Autodesk Inventor part; units mm, degrees
ref_plane "XZ Plane" through (0, 0, 0) normal (0, 1, 0) x (-1, 0, 0)
ref_plane "XY Plane" through (0, 0, 0) normal (0, 0, 1) x (1, 0, 0)
sketch "Sketch1" plane through (0, 0, 0) normal (0, 1, 0) x (-1, 0, 0)
  line L0 (47.625, 50.8) -> (-47.625, 50.8)
  line L1 (-47.625, 50.8) -> (-47.625, -50.8)
  line L2 (-47.625, -50.8) -> (47.625, -50.8)
  line L3 (47.625, -50.8) -> (47.625, 50.8)
  line L4 (47.625, 50.8) -> (-47.625, -50.8) construction
  line L5 (-47.625, 50.8) -> (47.625, -50.8) construction
  point P0 (0, 0)
  dimension "d0" = 95.25
  dimension "d1" = 101.6
extrude "Extrusion1" add sketch "Sketch1" against normal blind 3.175
sketch "Sketch2" plane through (0, 0, 0) normal (0, 1, 0) x (1, 0, 0)
  line L0 (-47.625, -19.05) -> (-28.575, -19.05)
  line L1 (-28.575, -19.05) -> (-28.575, 19.05)
  line L2 (-28.575, 19.05) -> (-47.625, 19.05)
  line L3 (-47.625, 19.05) -> (-47.625, -19.05)
  line L4 (-47.625, -19.05) -> (-28.575, 19.05) construction
  line L5 (-28.575, -19.05) -> (-47.625, 19.05) construction
  line L6 (-44.45, -15.875) -> (-31.75, -15.875)
  line L7 (-31.75, -15.875) -> (-31.75, 15.875)
  line L8 (-31.75, 15.875) -> (-44.45, 15.875)
  line L9 (-44.45, 15.875) -> (-44.45, -15.875)
  line L10 (-44.45, -15.875) -> (-31.75, 15.875) construction
  line L11 (-31.75, -15.875) -> (-44.45, 15.875) construction
  line L12 (-47.625, 50.8) -> (47.625, 50.8) construction
  line L13 (0, 50.8) -> (0, -101.6) construction
  line L14 (47.625, -19.05) -> (28.575, -19.05)
  line L15 (28.575, -19.05) -> (28.575, 19.05)
  line L16 (28.575, 19.05) -> (47.625, 19.05)
  line L17 (47.625, 19.05) -> (47.625, -19.05)
  line L18 (44.45, -15.875) -> (31.75, -15.875)
  line L19 (31.75, -15.875) -> (31.75, 15.875)
  line L20 (31.75, 15.875) -> (44.45, 15.875)
  line L21 (44.45, 15.875) -> (44.45, -15.875)
  point P0 (0, 0)
  point P1 (-38.1, 0)
  dimension "d4" = 38.1
  dimension "d5" = 19.05
  dimension "d6" = 38.1
  dimension "d7" = 3.175
  dimension "d8" = 3.175
extrude "Extrusion2" add sketch "Sketch2" along normal blind 101.6
sketch "Sketch4" plane through (-47.625, -3.175, -50.8) normal (-1, 0, 0) x (0, 0, 1)
  line L0 (50.8, 3.175) -> (50.8, 93.283) construction
  circle A0 centre (50.8, 79.375) radius 4.7625
  line L1 (0, 3.175) -> (31.75, 3.175)
  dimension "d15" = 9.525
  dimension "d16" = 76.2
extrude "Extrusion4" cut sketch "Sketch4" against normal through all
equation "\"d0\" = BaseWidth"
equation "\"d1\" = BaseLength"
equation "\"d2\" = BaseThickness"
equation "\"d5\" = postWidth"
equation "\"d6\" = postLength"
equation "\"d7\" = postThickness"
equation "\"d8\" = postThickness"
equation "\"d9\" = postHeight"
equation "\"d15\" = axelDiam"
equation "\"d16\" = axelHeightAbovePlate"
equation "\"BaseWidth\" = 95.25"
equation "\"BaseLength\" = 101.6"
equation "\"BaseThickness\" = 3.175"
equation "\"postWidth\" = 19.05"
equation "\"postLength\" = 38.1"
equation "\"postThickness\" = 3.175"
equation "\"postCenterDistanceFromCenterOfBase\" = 38.1"
equation "\"axelDiam\" = 9.525"
equation "\"axelHeightAbovePlate\" = 76.2"
properties part number "PostForLift"
The listing builds one solid part. Answer for the finished solid, in the listing's coordinates (mm). A direction names the side the tool comes from. Coordinates: 2 decimals unless noted, no trailing zeros. Loops run counter-clockwise (first coordinate to the right, second up) from the corner with the lowest first, then second, coordinate; pieces in that order, holes last. Notation, with made-up numbers: M 45.5,-0.75 L 69.5,-0.75 A22 cw 69.5,16.25 Z; hole C -38.5,67.5 d10. An arc over 180 degrees is marked long. Answer as CSV lines item,"result". Start each with the question number.
(1) For faces 1 (the flat face through (-38, 50, 15.875)), 2 (the cylindrical face through (30.14, 80.92, -0.62)), 3 (the flat face through (-47.625, 42, 4)), 4 (the flat face through (-38, 50, 19.05)), 5 (the flat face through (-28.575, 50, 0)), determine the directions among +Z, -Z, +X, -X, +Y, -Y from which every point of the face is accessible in a straight line to the end or side of a thin tool.
(2) The part is cut by section B-B (z = 0). State how many separate pieces and enclosed holes the cut face has, and give its area (3 significant figures).
(3) Given pin 1 (2 mm diameter, centred on y = 7.5, z = -22, fed in from +X); pin 2 (6.5 mm diameter, centred on x = 38, z = 0, fed in from +Y); pin 3 (15 mm diameter, centred on x = 36.5, y = 63, fed in from +Z); pin 4 (15 mm diameter, centred on x = 37, y = 40, fed in from -Z), each flat-ended and moving along its own axis, determine where each tip first touches the part or whether it passes through.
(4) The part is cut by section D-D (x = 12). Give the vertices of the cut face in (y, z) (3 decimals), and give its area (3 significant figures).
(5) Find the intervals of material crossed by L1, parallel to X at y = 4.5, z = 12 (3 decimals); L2, parallel to Y at x = -30.7, z = 0 (1 decimal); L3, parallel to Z at x = -30, y = 76, in increasing order. Write a range as [from, to].
(6) The mould has two halves that part along Z. Classify faces 6 (the flat face through (38, 50, -19.05)), 7 (the flat face through (-38, 0, 0)), 8 (the flat face through (38, 50, 19.05)): pulls with the +Z half, pulls with the -Z half, needs draft (parallel to the pull), parting line crosses it, or undercut.
(7) The part is cut by section A-A (y = 56.5). Give the vertices of the cut face in (x, z) (3 decimals), and give its area (3 significant figures).
Determined:
1,face 1,"+Y"
1,face 2,"+X, -X"
1,face 3,"+Z, -Z, -X, +Y, -Y"
1,face 4,"+Z, +X, -X, +Y"
1,face 5,"+Z, -Z, +Y"
2,separate pieces,"5"
2,enclosed holes,"0"
2,area,"1,470 mm2"
3,pin 1,"through"
3,pin 2,"y = 0"
3,pin 3,"z = 19.05"
3,pin 4,"z = -19.05"
4,outline,"M -3.175,-50.8 L 0,-50.8 L 0,50.8 L -3.175,50.8 Z"
4,area,"323 mm2"
5,L1,"[-47.625, -44.45], [-31.75, -28.575], [28.575, 31.75], [44.45, 47.625]"
5,L2,"[-3.2, 71.4], [81, 101.6]"
5,L3,"[-19.05, -4.76], [4.76, 19.05]"
6,face 6,"pulls with the -Z half"
6,face 7,"undercut"
6,face 8,"pulls with the +Z half"
7,outline,"M -47.625,-19.05 L -28.575,-19.05 L -28.575,19.05 L -47.625,19.05 Z; M 28.575,-19.05 L 47.625,-19.05 L 47.625,19.05 L 28.575,19.05 Z; hole M -44.45,-15.875 L -31.75,-15.875 L -31.75,15.875 L -44.45,15.875 Z; hole M 31.75,-15.875 L 44.45,-15.875 L 44.45,15.875 L 31.75,15.875 Z"
7,area,"645 mm2"
